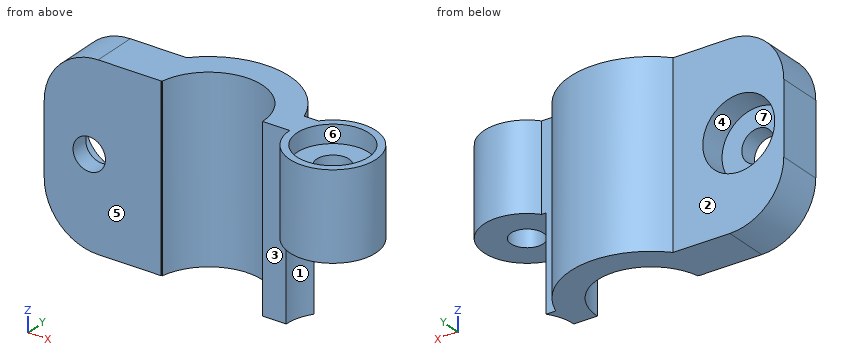
```python
from build123d import *

# Parameters (mm, degrees)
CYLINDER095_R     = 4
CYLINDER095_DEPTH = 20
CYLINDER096_R     = 4
CYLINDER096_DEPTH = 2
CYLINDER005_R     = 5.2
CYLINDER005_DEPTH = 10.4
CYLINDER003_R     = 1.8
CYLINDER003_DEPTH = 50
CYLINDER001_W     = 6
CYLINDER001_H     = 20
CYLINDER001_ANGLE = 180
CYLINDER004_R     = 1.8
CYLINDER004_DEPTH = 20
BOX_W             = 13
BOX_H             = 5
BOX_DEPTH         = 20
FILLET_R          = 6
CYLINDER002_R     = 4.8
CYLINDER002_DEPTH = 20
CYLINDER_W        = 9
CYLINDER_H        = 20
CYLINDER_ANGLE    = 170
BOX001_W          = 7.8
BOX001_H          = 3
BOX001_DEPTH      = 20


with BuildPart() as bolt_head_cylinder:
    # Cylinder095 → Cylinder095 (new body)
    with BuildSketch(Plane(origin=(-14, 3, 10), x_dir=(1, 0, 0), z_dir=(0, 1, 0))):
        Circle(CYLINDER095_R)
    extrude(amount=CYLINDER095_DEPTH)


with BuildPart() as bolt_head_side_cylinder:
    # Cylinder096 → Cylinder096 (new body)
    with BuildSketch(Plane(origin=(13.8, 0, 18), x_dir=(1, 0, 0), z_dir=(0, 0, 1))):
        Circle(CYLINDER096_R)
    extrude(amount=CYLINDER096_DEPTH)


with BuildPart() as top_half_remove_fusion:
    # Cylinder005 → Cylinder005 (new body)
    with BuildSketch(Plane(origin=(13.8, 0, 0), x_dir=(1, 0, 0), z_dir=(0, 0, 1))):
        Circle(CYLINDER005_R)
    extrude(amount=CYLINDER005_DEPTH)

    # Fusion002: union bolt head cylinder, bolt head side cylinder
    add(bolt_head_cylinder.part)
    add(bolt_head_side_cylinder.part)


with BuildPart() as bolt_hole:
    # Cylinder003 → Cylinder003 (new body)
    with BuildSketch(Plane(origin=(-14, 20, 10), x_dir=(1, 0, 0), z_dir=(0, -1, 0))):
        Circle(CYLINDER003_R)
    extrude(amount=CYLINDER003_DEPTH)


with BuildPart() as hole_cylinder:
    # Cylinder001 → Cylinder001 (revolve)
    with BuildSketch(Plane.XZ):
        with Locations((3, 10)):
            Rectangle(CYLINDER001_W, CYLINDER001_H)
    revolve(axis=Axis((0, 0, 0), (0, 0, 1)), revolution_arc=CYLINDER001_ANGLE)


with BuildPart() as hole_fusion:
    # Cylinder004 → Cylinder004 (new body)
    with BuildSketch(Plane(origin=(13.8, 0, 0), x_dir=(1, 0, 0), z_dir=(0, 0, 1))):
        Circle(CYLINDER004_R)
    extrude(amount=CYLINDER004_DEPTH)

    # Fusion: union bolt hole, hole cylinder
    add(bolt_hole.part)
    add(hole_cylinder.part)


with BuildPart() as petal_fillet:
    # Box → Box (new body)
    with BuildSketch(Plane(origin=(-19, 1, 0), x_dir=(1, 0, 0), z_dir=(0, 0, 1))):
        with Locations((6.5, 2.5)):
            Rectangle(BOX_W, BOX_H)
    extrude(amount=BOX_DEPTH)

    # Fillet
    fillet_edges = [petal_fillet.edges().sort_by_distance(p)[0] for p in [
        (-19, 3.5, 20),
        (-19, 3.5, 0),
    ]]
    fillet(fillet_edges, radius=FILLET_R)


with BuildPart() as side_cylinder:
    # Cylinder002 → Cylinder002 (new body)
    with BuildSketch(Plane(origin=(13.8, 0, 0), x_dir=(1, 0, 0), z_dir=(0, 0, 1))):
        Circle(CYLINDER002_R)
    extrude(amount=CYLINDER002_DEPTH)


with BuildPart() as external_cylinder:
    # Cylinder → Cylinder (revolve)
    with BuildSketch(Plane.XZ):
        with Locations((4.5, 10)):
            Rectangle(CYLINDER_W, CYLINDER_H)
    revolve(axis=Axis((0, 0, 0), (0, 0, 1)), revolution_arc=CYLINDER_ANGLE)


with BuildPart() as top_half_clone:
    # Box001 → Box001 (new body)
    with BuildSketch(Plane(origin=(6, 0, 0), x_dir=(1, 0, 0), z_dir=(0, 0, 1))):
        with Locations((3.9, 1.5)):
            Rectangle(BOX001_W, BOX001_H)
    extrude(amount=BOX001_DEPTH)

    # Fusion001: union petal fillet, side cylinder, external cylinder
    add(petal_fillet.part)
    add(side_cylinder.part)
    add(external_cylinder.part)

    # Cut: cut hole fusion
    add(hole_fusion.part, mode=Mode.SUBTRACT)

    # Cut001: cut top half remove fusion
    add(top_half_remove_fusion.part, mode=Mode.SUBTRACT)


solid = top_half_clone.part
```
Part model, mm, in its own coordinate system. Face numbers are marked on the shaded views. A direction names the side the tool comes from. Round coordinates to 2 decimals unless told otherwise and drop trailing zeros. Write each loop counter-clockwise with the first axis right and the second up, starting at its lowest first coordinate (ties: lowest second). Pieces come first, ordered by that corner, then holes. Notation, with made-up numbers: (51, -28) -> (95, -28) arc R33 cw to (95, 1) -> close; hole circle Ø8 at (52.25, -15). An arc over 180 degrees is marked (long way). Return JSON: item names as keys, results as strings. Group by question number.
Q1. Pin check, flat tips, straight feed: pin 1 (10.5 mm diameter, centred on x = -13.5, z = 6, fed in from -Y); pin 2 (6 mm diameter, centred on x = -14, z = 6.5, fed in from +Y); pin 3 (1.5 mm diameter, centred on x = 10, z = 12.5, fed in from -Y); pin 4 (1.5 mm diameter, centred on x = 7, y = 6.5, fed in from -Z). Stop position of each tip, or through.
Q2. Saw through at C-C on y = -1. Write the cut outline in (x, z).
Q3. Saw through at A-A on z = 10. Write the cut outline in (x, y).
Q4. Mould opens along Y. For the marked faces 5, 6 and 7 say: pulls with the +Y half, pulls with the -Y half, needs draft (parallel to the pull), parting line crosses it, or undercut.
Q5. Saw through at D-D on y = 2.5. Write the cut outline in (x, z).
Q6. Which spindle directions (+Z, -Z, +X, -X, +Y, -Y) get a long thin tool onto all of the face, cutting with end or side? Do the marked faces 1, 2, 3 and 4. Say none if no direction does.
Q7. Saw through at B-B on x = -14. Write the cut outline in (y, z).
Q8. Probe L1, parallel to Y at x = 13.8, z = 19.3; L2, parallel to X at y = 1.7, z = 10; L3, parallel to Y at x = 13.8, z = 14.5. List the from-to ranges inside material, lowest first. Write a range as [from, to].
Answer:
{
 "1": {"pin 1": "y = 1", "pin 2": "y = 6", "pin 3": "y = -3.71", "pin 4": "z = 0"},
 "2": {"outline": "(9.11, 10.4) -> (12.3, 10.4) -> (12.3, 18) -> (9.93, 18) -> (9.93, 20) -> (9.11, 20) -> close; (15.3, 10.4) -> (18.49, 10.4) -> (18.49, 20) -> (17.67, 20) -> (17.67, 18) -> (15.3, 18) -> close"},
 "3": {"outline": "(-19, 1) -> (-15.8, 1) -> (-15.8, 3) -> (-18, 3) -> (-18, 6) -> (-19, 6) -> close; (-12.2, 1) -> (-6, 1) -> (-6, 1.06) -> (-5.91, 1.04) arc R6 cw to (6, 0) -> (8.6, 0) arc R5.2 cw to (9.55, 3) -> (8.49, 3) arc R9 ccw to (-6.71, 6) -> (-10, 6) -> (-10, 3) -> (-12.2, 3) -> close"},
 "4": {"face 5": "pulls with the -Y half", "face 6": "undercut", "face 7": "pulls with the +Y half"},
 "5": {"outline": "(-19, 6) arc R6 ccw to (-13, 0) -> (-5.45, 0) -> (-5.45, 20) -> (-13, 20) arc R6 ccw to (-19, 14) -> close; (5.45, 0) -> (9.24, 0) -> (9.24, 10.4) -> (17.9, 10.4) -> (17.9, 20) -> (16.92, 20) -> (16.92, 18) -> (10.68, 18) -> (10.68, 20) -> (5.45, 20) -> close; hole circle Ø3.6 at (-14, 10)"},
 "6": {"face 1": "-Z, +X, -Y", "face 2": "+Z, -Z, -X, +Y", "face 3": "+Z, -Z, -X, -Y", "face 4": "+Y"},
 "7": {"outline": "(1, 0.08) -> (6, 0.08) -> (6, 6) -> (3, 6) -> (3, 8.2) -> (1, 8.2) -> close; (1, 11.8) -> (3, 11.8) -> (3, 14) -> (6, 14) -> (6, 19.92) -> (1, 19.92) -> close"},
 "8": {"L1": "[-4.8, -4], [4, 4.8]", "L2": "[-19, -15.8], [-12.2, -5.75], [5.75, 8.89]", "L3": "[-4.8, -1.8], [1.8, 4.8]"}
}
